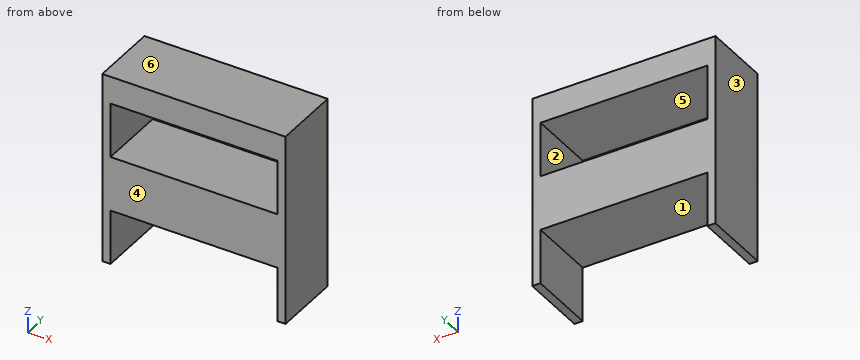
```python
from build123d import *

# Parameters (mm, degrees)
F0_W     = 61
F0_H     = 20
F1_DEPTH = 25


with BuildPart() as f1:
    # F0 (on Front) → F1 (new body)
    with BuildSketch(Plane.XZ):
        Polygon((-14.266822, 0.092322), (-11.266822, 0.092322), (-11.266822, 20.092322), (-11.266822, 40.092322), (-11.266822, 60.092322), (49.733178, 60.092322), (49.733178, 40.092322), (49.733178, 20.092322), (49.733178, 0.092322), (52.733178, 0.092322), (52.733178, 70.092322), (49.733178, 70.092322), (-14.266822, 70.092322), align=None)
        with Locations((19.233178, 30.092322)):
            Rectangle(F0_W, F0_H)
    extrude(amount=F1_DEPTH)


solid = f1.part
```
The model under review builds one solid part; all positions refer to its coordinate system, in mm. Face numbers are marked on the shaded views. A direction names the side the tool comes from. Round coordinates to 2 decimals unless told otherwise and drop trailing zeros. Write each loop counter-clockwise with the first axis right and the second up, starting at its lowest first coordinate (ties: lowest second). Pieces come first, ordered by that corner, then holes.
(1) Wall thickness on L1, parallel to Z at x = 33, y = -10.5; L2, parallel to X at y = -5, z = 53: over which ranges is each line inside the solid? List them lowest first.
(2) We need section A-A on x = 16. Give the boundary of the cut face in (y, z).
(3) We need section B-B on z = 53.5. Give the boundary of the cut face in (x, y).
(4) Mouldability with a two-part tool opening along Z and no side actions: class the marked faces 4, 5 and 6 as +Z half, -Z half, draft (parallel to the pull), parting line (faces both ways), or undercut.
(5) Machinability: for the marked faces 1, 2 and 3, which of the approach directions +Z, -Z, +X, -X, +Y, -Y give a long, thin tool a straight path to every point of the face, cutting with its end or side? Answer none if there is none.
(6) Insertion check: pin 1 (2 mm diameter, centred on x = 8.5, z = 33, fed in from +Y); pin 2 (12 mm diameter, centred on x = 40.5, y = -14.5, fed in from -Z). Each pin has a flat end and moves straight along its axis. Give the tip position at first contact, or say it passes through.
(7) We need section C-C on y = -19. Give the boundary of the cut face in (x, z), and give its area (3 significant figures).
Findings below:
1. L1: z = 20.09 to 40.09, 60.09 to 70.09
1. L2: x = -14.27 to -11.27, 49.73 to 52.73
2. outline: (-25, 20.09) - (0, 20.09) - (0, 40.09) - (-25, 40.09) - close; (-25, 60.09) - (0, 60.09) - (0, 70.09) - (-25, 70.09) - close
3. outline: (-14.27, -25) - (-11.27, -25) - (-11.27, 0) - (-14.27, 0) - close; (49.73, -25) - (52.73, -25) - (52.73, 0) - (49.73, 0) - close
4. face 4: draft
4. face 5: undercut
4. face 6: +Z half
5. face 1: -Z, +Y, -Y
5. face 2: +Y, -Y
5. face 3: +Z, -Z, -X, +Y, -Y
6. pin 1: stops at y = 0
6. pin 2: stops at z = 20.09
7. outline: (-14.27, 0.09) - (-11.27, 0.09) - (-11.27, 20.09) - (49.73, 20.09) - (49.73, 0.09) - (52.73, 0.09) - (52.73, 70.09) - (-14.27, 70.09) - close; hole (-11.27, 40.09) - (49.73, 40.09) - (49.73, 60.09) - (-11.27, 60.09) - close
7. area: 2,250 mm2
